The drawing under review shows one solid part. Ordinate dimensions are in mm from its lowest x, y, z. A direction names the side the tool comes from. Coordinates: 2 decimals unless noted, no trailing zeros. Order: outer loops, then holes, each group sorted by start corner. A loop starts at its lowest first (then second) coordinate and runs counter-clockwise, first axis right, second up.
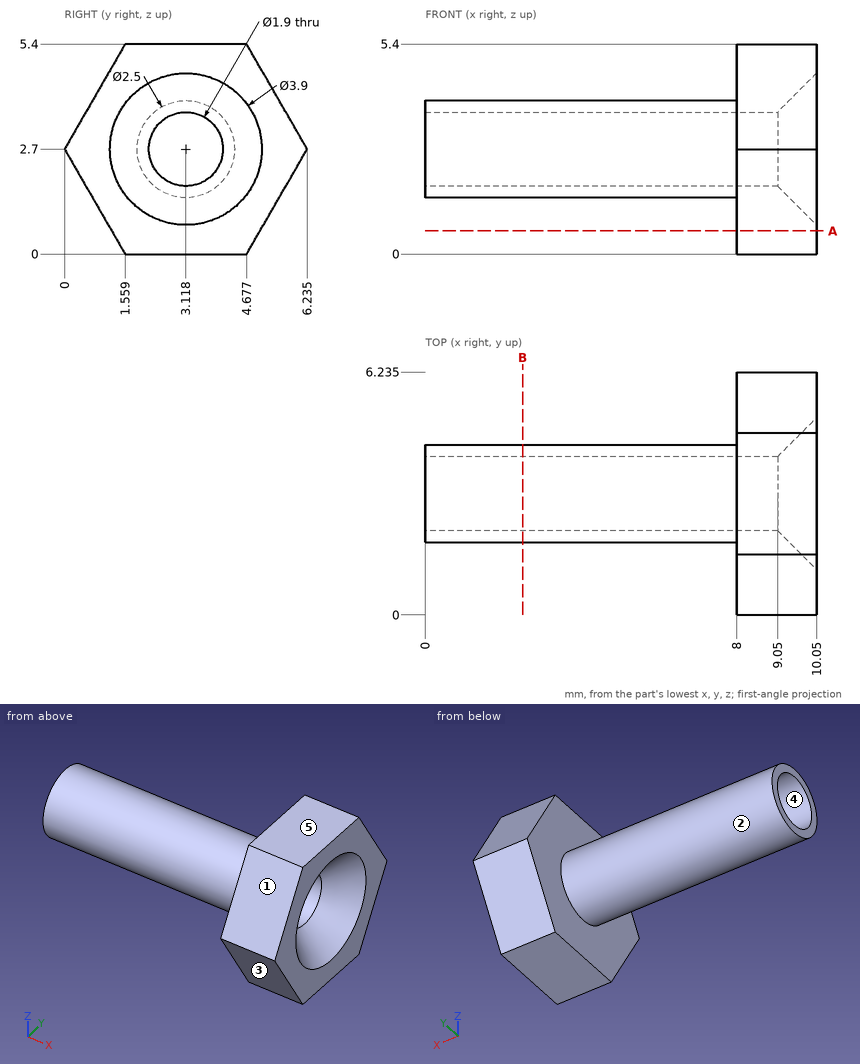
1. To check wall thickness, follow line 1 (Y direction, x = 4.75, z = 2.7); line 2 (X direction, y = 5.5, z = 2.9); line 3 (Z direction, x = 9.5, y = 2) (1 decimal). State the ranges of each line that lie inside material, in increasing order.
2. Mouldability with a two-part tool opening along Y and no side actions: class the marked faces 3, 4 and 5 as pulls with the +Y half, pulls with the -Y half, needs draft (parallel to the pull), parting line crosses it, or undercut.
3. Add section A-A (z = 0.6). Give the boundary of the cut face in (x, y).
4. For the marked faces 1 and 2, list the 3-axis set-ups (+Z, -Z, +X, -X, +Y, -Y) from which the entire face can be reached by the end or side of a thin tool; tool diameter is ignored.
5. Add section B-B (x = 2.5). Give the boundary of the cut face in (y, z).
6. Insertion check: pin 1 (2 mm diameter, centred on x = 4.5, y = 5, fed in from -Z) (1 decimal); pin 2 (1.5 mm diameter, centred on x = 4.5, z = 1.5, fed in from +Y); pin 3 (1.6 mm diameter, centred on y = 3.5, z = 2.5, fed in from -X). Each pin has a flat end and moves straight along its axis. Give the tip position at first contact, or say it passes through.
Solution:
1. line 1: y = 1.87 to 2.17, 4.07 to 4.37
1. line 2: x = 8 to 10.05
1. line 3: z = 0 to 1.9, 3.5 to 5.4
2. face 3: pulls with the -Y half
2. face 4: undercut
2. face 5: needs draft
3. outline: (8, 1.21) - (10.05, 1.21) - (10.05, 5.02) - (8, 5.02) - close
4. face 1: +Z, +X, -X, -Y
4. face 2: -X
5. outline: circle Ø2.5 at (3.12, 2.7); hole circle Ø1.9 at (3.12, 2.7)
6. pin 1: stops at z = 1.8
6. pin 2: stops at y = 4.28
6. pin 3: stops at x = 0
